Input: part model. Units: mm. Frame: model coordinates. A direction names the side the tool comes from. Coordinates: 2 decimals unless noted, no trailing zeros. Write each loop counter-clockwise with the first axis right and the second up, starting at its lowest first coordinate (ties: lowest second). Pieces come first, ordered by that corner, then holes. Notation, with made-up numbers: (38, -39.5) - (89, -39.5) arc R24 ccw to (89, -0.5) - close; hole circle Ø5 at (-31.5, 51.25). An arc over 180 degrees is marked (long way). Put each result on its own line as item: value. Start each with the question number.
1. Cut plane B-B, the plane y = 152. Return loops of the section in (x, z).
2. Pull-direction query (X, two-part tool) for faces 3 (the flat face through (15, 249, -7)), 4 (the flat face through (7, 249, -13.5)), 5 (the flat face through (0, 249, -7)), 6 (the flat face through (7, 249, -1.5)); classes: released by +X, released by -X, zero draft, split by the parting line, or undercut.
3. Cut plane A-A, the plane x = 8. Return loops of the section in (y, z).
4. Pin query (flat end, axial travel): pin 1 (3 mm diameter, centred on x = 4, y = 235.5, fed in from +Z); pin 2 (3.5 mm diameter, centred on y = 10, z = -7.5, fed in from -X). Return the tip coordinate at first contact, or that it passes through.
5. Access query for faces 1 (the flat face through (14, 506, -8)), 2 (the flat face through (13.5, 249, -7)). Directions: +Z, -Z, +X, -X, +Y, -Y. A direction counts if a zero-diameter tool reaches every point of the face in a straight line with its end or side. Return the directions, or none.
6. Line query: line 1 (Y direction, x = 14.25, z = -7.5); line 2 (X direction, y = 262.5, z = -9); line 3 (Z direction, x = 8, y = 126). Output: solid intervals per line, ascending.
from build123d import *

# Parameters (mm, degrees)
SKETCH_1_W          = 15
SKETCH_1_H          = 15
SKETCH_1_W_2        = 12
SKETCH_1_H_2        = 12
EXTRUDE_1_DEPTH     = 506
CUT_EXTRUDE_1_REACH = 508.444
SKETCH_2_R          = 2.6
SKETCH_2_R_2        = 2.15


with BuildPart() as part:
    # ｽｹｯﾁ1 → 押し出し-薄板1 (new body)
    with BuildSketch(Plane(origin=(0, 0, 0), x_dir=(1, 0, 0), z_dir=(0, 1, 0))):
        with Locations((7.5, 7.5)):
            Rectangle(SKETCH_1_W, SKETCH_1_H)
        with Locations((7.5, 7.5)):
            Rectangle(SKETCH_1_W_2, SKETCH_1_H_2, mode=Mode.SUBTRACT)
    extrude(amount=EXTRUDE_1_DEPTH)

    # ｶｯﾄ - 押し出し1: up to this face of the body (flat: up to its plane)
    cut_extrude_1_end = Plane(part.part.faces().sort_by_distance((0, 253, -7.5))[0])
    # ｽｹｯﾁ2 → ｶｯﾄ - 押し出し1 (cut, up to the picked face)
    with BuildSketch(Plane(origin=(15, 0, 0), x_dir=(0, 0, -1), z_dir=(1, 0, 0)), mode=Mode.PRIVATE) as cut_extrude_1_sk1:
        with Locations((7.5, 496)):
            Circle(SKETCH_2_R)
    cut_extrude_1_tool1 = split(extrude(cut_extrude_1_sk1.sketch, amount=-CUT_EXTRUDE_1_REACH, mode=Mode.PRIVATE), bisect_by=cut_extrude_1_end, keep=Keep.BOTH, mode=Mode.PRIVATE)
    # ｽｹｯﾁ2 → ｶｯﾄ - 押し出し1 (cut, up to the picked face)
    with BuildSketch(Plane(origin=(15, 0, 0), x_dir=(0, 0, -1), z_dir=(1, 0, 0)), mode=Mode.PRIVATE) as cut_extrude_1_sk2:
        with Locations((7.5, 10)):
            Circle(SKETCH_2_R_2)
    cut_extrude_1_tool2 = split(extrude(cut_extrude_1_sk2.sketch, amount=-CUT_EXTRUDE_1_REACH, mode=Mode.PRIVATE), bisect_by=cut_extrude_1_end, keep=Keep.BOTH, mode=Mode.PRIVATE)
    # ｽｹｯﾁ2 → ｶｯﾄ - 押し出し1 (cut, up to the picked face)
    with BuildSketch(Plane(origin=(15, 0, 0), x_dir=(0, 0, -1), z_dir=(1, 0, 0)), mode=Mode.PRIVATE) as cut_extrude_1_sk3:
        with Locations((7.5, 50)):
            Circle(SKETCH_2_R_2)
    cut_extrude_1_tool3 = split(extrude(cut_extrude_1_sk3.sketch, amount=-CUT_EXTRUDE_1_REACH, mode=Mode.PRIVATE), bisect_by=cut_extrude_1_end, keep=Keep.BOTH, mode=Mode.PRIVATE)
    # ｽｹｯﾁ2 → ｶｯﾄ - 押し出し1 (cut, up to the picked face)
    with BuildSketch(Plane(origin=(15, 0, 0), x_dir=(0, 0, -1), z_dir=(1, 0, 0)), mode=Mode.PRIVATE) as cut_extrude_1_sk4:
        with Locations((7.5, 96)):
            Circle(SKETCH_2_R)
    cut_extrude_1_tool4 = split(extrude(cut_extrude_1_sk4.sketch, amount=-CUT_EXTRUDE_1_REACH, mode=Mode.PRIVATE), bisect_by=cut_extrude_1_end, keep=Keep.BOTH, mode=Mode.PRIVATE)
    add(cut_extrude_1_tool1.solids().sort_by(Axis((15, 496, -7.5), (-1, 0, 0)))[0], mode=Mode.SUBTRACT)
    add(cut_extrude_1_tool2.solids().sort_by(Axis((15, 10, -7.5), (-1, 0, 0)))[0], mode=Mode.SUBTRACT)
    add(cut_extrude_1_tool3.solids().sort_by(Axis((15, 50, -7.5), (-1, 0, 0)))[0], mode=Mode.SUBTRACT)
    add(cut_extrude_1_tool4.solids().sort_by(Axis((15, 96, -7.5), (-1, 0, 0)))[0], mode=Mode.SUBTRACT)


solid = part.part
Report:
1. outline: (0, -15) - (15, -15) - (15, 0) - (0, 0) - close; hole (1.5, -13.5) - (13.5, -13.5) - (13.5, -1.5) - (1.5, -1.5) - close
2. face 3: released by +X
2. face 4: undercut
2. face 5: released by -X
2. face 6: undercut
3. outline: (0, -15) - (506, -15) - (506, -13.5) - (0, -13.5) - close; (0, -1.5) - (506, -1.5) - (506, 0) - (0, 0) - close
4. pin 1: stops at z = 0
4. pin 2: passes through
5. face 1: +Z, -Z, +X, -X, +Y
5. face 2: +Y, -Y
6. line 1: y = 0 to 7.85, 12.15 to 47.85, 52.15 to 93.4, 98.6 to 493.4, 498.6 to 506
6. line 2: x = 0 to 1.5, 13.5 to 15
6. line 3: z = -15 to -13.5, -1.5 to 0
